from build123d import *

# Parameters (mm, degrees)
SKETCH1_W           = 11.5
SKETCH1_H           = 66.675
SKETCH1_W_2         = 3.175
BOSS_EXTRUDE1_DEPTH = 3.175


with BuildPart() as part:
    # Sketch1 → Boss-Extrude1 (new body)
    with BuildSketch(Plane(origin=(0, 0, 0), x_dir=(1, 0, 0), z_dir=(0, 1, 0))):
        Polygon((-52.96, 85.881432482), (52.96, 85.881432482), (52.96, 82.706432482), (65.66, 82.706432482), (65.66, -72.868567518), (62.485, -72.868567518), (62.485, -85.568567518), (-62.485, -85.568567518), (-62.485, -72.868567518), (-65.66, -72.868567518), (-65.66, 82.706432482), (-52.96, 82.706432482), align=None)
        Polygon((-52.96, 6.506432482), (-14.097750884, 6.506432482), (-52.96, 62.098375408), align=None, mode=Mode.SUBTRACT)
        Polygon((-45.212249116, 73.181432482), (-6.35, 73.181432482), (-6.35, 17.589489555), align=None, mode=Mode.SUBTRACT)
        with Locations((-34.0045, -39.531067518)):
            Rectangle(SKETCH1_W, SKETCH1_H, mode=Mode.SUBTRACT)
        Polygon((52.96, 62.098375408), (52.96, 6.506432482), (14.097750884, 6.506432482), align=None, mode=Mode.SUBTRACT)
        Polygon((6.35, 73.181432482), (6.35, 17.589489555), (45.212249116, 73.181432482), align=None, mode=Mode.SUBTRACT)
        Polygon((14.097750884, -6.193567518), (52.96, -6.193567518), (52.96, -61.785510445), align=None, mode=Mode.SUBTRACT)
        Polygon((6.35, -17.276624592), (45.212249116, -72.868567518), (6.35, -72.868567518), align=None, mode=Mode.SUBTRACT)
        with Locations((-7.9375, -39.531067518)):
            Rectangle(SKETCH1_W_2, SKETCH1_H, mode=Mode.SUBTRACT)
    extrude(amount=BOSS_EXTRUDE1_DEPTH)


solid = part.part
For this review, take the finished solid that the model builds, in its own axes (mm). A direction names the side the tool comes from. Coordinates: 2 decimals unless noted, no trailing zeros. Loops run counter-clockwise (first coordinate to the right, second up) from the corner with the lowest first, then second, coordinate; pieces in that order, holes last. Notation, with made-up numbers: (-2.5, -20) -> (11.5, -20) arc R10 ccw to (11.5, -14) -> close; hole circle Ø10 at (67.5, 84.5). An arc over 180 degrees is marked (long way). Write each question's results on one line, items separated by ' | '.
Q1. Machinability: for faces 3 (the flat face through (1, 0, -1)), 4 (the flat face through (33.257, 1.565, -33.913)), which of the approach directions +Z, -Z, +X, -X, +Y, -Y give a long, thin tool a straight path to every point of the face, cutting with its end or side? Answer none if there is none.
Taken from the geometry:
face 3: +Z, -Z, +X, -X, -Y | face 4: +Y, -Y
Q2. Add section A-A, the plane z = -68.5. State the section outline as (x, y) points (3 decimals).
Taken from the geometry:
outline: (-65.66, 0) -> (-41.94, 0) -> (-41.94, 3.175) -> (-65.66, 3.175) -> close; (-6.35, 0) -> (6.35, 0) -> (6.35, 3.175) -> (-6.35, 3.175) -> close; (41.94, 0) -> (65.66, 0) -> (65.66, 3.175) -> (41.94, 3.175) -> close
Q3. To check wall thickness, follow line 1 along Z through (x, y) = (-37.5, 2.35); line 2 along Z through (x, y) = (-18, 2.15); line 3 along X through (y, z) = (2.1, -30.5). State the ranges of each line that lie inside material, in increasing order. Write a range as [from, to].
Taken from the geometry:
line 1: [-85.88, -73.18], [-62.15, -39.98], [-6.51, 6.19], [72.87, 85.57] | line 2: [-85.88, -73.18], [-34.25, -12.09], [-6.51, 85.57] | line 3: [-65.66, -52.96], [-30.87, -15.38], [-6.35, 6.35], [15.38, 30.87], [52.96, 65.66]
Q4. Mouldability with a two-part tool opening along Z and no side actions: class faces 1 (the flat face through (-25.51, 1.57, -45)), 2 (the flat face through (1, 3.175, -1)) as +Z half, -Z half, draft (parallel to the pull), parting line (faces both ways), or undercut.
Taken from the geometry:
face 1: undercut | face 2: draft
Q5. For pin 1 Ø1.6 at (y, z) = (1, 76) entering from +X (3 decimals); pin 2 Ø1 at (x, z) = (-7.5, 7) entering from +Y; pin 3 Ø1 at (y, z) = (2, -84) entering from +X, all flat-tipped, find the tip position at first contact; note any pin that passes through.
Taken from the geometry:
pin 1: x = 62.485 | pin 2: through | pin 3: x = 52.96
Q6. Add section B-B, the plane x = -42.5. State the section outline as (y, z) points (3 decimals).
Taken from the geometry:
outline: (0, -85.881) -> (3.175, -85.881) -> (3.175, -73.181) -> (0, -73.181) -> close; (0, -69.302) -> (3.175, -69.302) -> (3.175, -47.135) -> (0, -47.135) -> close; (0, -6.506) -> (3.175, -6.506) -> (3.175, 85.569) -> (0, 85.569) -> close
Q7. Add section C-C, the plane z = -51. State the section outline as (x, y) points (3 decimals).
Taken from the geometry:
outline: (-65.66, 0) -> (-52.96, 0) -> (-52.96, 3.175) -> (-65.66, 3.175) -> close; (-45.202, 0) -> (-29.706, 0) -> (-29.706, 3.175) -> (-45.202, 3.175) -> close; (-6.35, 0) -> (6.35, 0) -> (6.35, 3.175) -> (-6.35, 3.175) -> close; (29.706, 0) -> (45.202, 0) -> (45.202, 3.175) -> (29.706, 3.175) -> close; (52.96, 0) -> (65.66, 0) -> (65.66, 3.175) -> (52.96, 3.175) -> close
Q8. Add section D-D, the plane x = 21.5. State the section outline as (y, z) points (1 decimal).
Taken from the geometry:
outline: (0, -85.9) -> (3.2, -85.9) -> (3.2, -73.2) -> (0, -73.2) -> close; (0, -39.3) -> (3.2, -39.3) -> (3.2, -17.1) -> (0, -17.1) -> close; (0, -6.5) -> (3.2, -6.5) -> (3.2, 6.2) -> (0, 6.2) -> close; (0, 16.8) -> (3.2, 16.8) -> (3.2, 38.9) -> (0, 38.9) -> close; (0, 72.9) -> (3.2, 72.9) -> (3.2, 85.6) -> (0, 85.6) -> close
